from build123d import *

# Parameters (mm, degrees)
F0_R        = 7.5
F1_DEPTH    = 20
F0_W        = 45
F0_H        = 45
F2_DEPTH    = 5
F3_R        = 2.5
F4_DEPTH    = 25
F5_R        = 10
F5_R_2      = 7.5
F6_DEPTH    = 7
F7_W        = 8
F7_H        = 9.7702028193
F7_W_2      = 5
F7_H_2      = 4.5
F8_DEPTH    = 2
F9_T3_DEPTH = 70
F9_T5_DEPTH = 70


# Not quite as in the source:
# - a fillet or chamfer that OpenCascade refuses, or shapes differently, is made with other operations: its cross-section is extruded or revolved along the edge and cut away or added


with BuildPart() as f1:
    # F0 (on Front) → F1 (new body)
    with BuildSketch(Plane.XZ):
        with Locations((-2.8196598027, -8.5107027553)):
            Circle(F0_R)
    extrude(amount=F1_DEPTH)

    # F0 (on Front) → F2 (join)
    with BuildSketch(Plane.XZ):
        with Locations((-2.8196598027, -8.5107027553)):
            Rectangle(F0_W, F0_H)
        with Locations((-2.8196598027, -8.5107027553)):
            Circle(F0_R, mode=Mode.SUBTRACT)
    extrude(amount=F2_DEPTH)

    # F3 (on face) → F4 (cut)
    with BuildSketch(Plane.XZ.offset(5)):
        with Locations((12.1803401973, 7.9892972447)):
            Circle(F3_R)
        with Locations((-17.8196598027, 7.9892972447)):
            Circle(F3_R)
    extrude(amount=-F4_DEPTH, mode=Mode.SUBTRACT)

    # F5 (on face) → F6 (join)
    with BuildSketch(Plane.XZ.offset(20)):
        with Locations((-2.8196598027, -8.5107027553)):
            Circle(F5_R)
        with Locations((-2.8196598027, -8.5107027553)):
            Circle(F5_R_2, mode=Mode.SUBTRACT)
        with Locations((-2.8196598027, -8.5107027553)):
            Circle(F5_R_2)
    extrude(amount=F6_DEPTH)

    # F7 (on face) → F8 (cut)
    with BuildSketch(Plane.XZ.offset(27)):
        with Locations((-2.8196598027, -15.6458041649)):
            Rectangle(F7_W, F7_H)
        with Locations((-9.3196598027, -8.5107027553)):
            Rectangle(F7_W_2, F7_H_2)
        with Locations((-2.8196598027, -8.5107027553)):
            Rectangle(F7_W, F7_H_2)
        with Locations((3.6803401973, -8.5107027553)):
            Rectangle(F7_W_2, F7_H_2)
        with Locations((-2.8196598027, -1.3756013457)):
            Rectangle(F7_W, F7_H)
    extrude(amount=-F8_DEPTH, mode=Mode.SUBTRACT)

    # F9: fillet of radius 5 on 7 edges, made by hand

    # F9_s1 → F9_t2 (revolve)
    with BuildSketch(Plane.XY.offset(-8.5107027553)):
        with BuildLine():
            ThreePointArc((4.6803401973, -10), (6.1448062914, -6.4644660941), (9.6803401973, -5))
            Line((9.6803401973, -5), (4.6803401973, -5))
            Line((4.6803401973, -5), (4.6803401973, -10))
        make_face()
    revolve(axis=Axis((-2.8196598027, -5, -8.5107027553), (0, -1, 0)))

    # F9_s4 → F9_t3 (cut)
    with BuildSketch(Plane.YZ.offset(-37.8196598027)):
        with BuildLine():
            ThreePointArc((-5, 8.9892972447), (-3.5355339059, 12.5248311506), (0, 13.9892972447))
            Line((0, 13.9892972447), (-5, 13.9892972447))
            Line((-5, 13.9892972447), (-5, 8.9892972447))
        make_face()
        with BuildLine():
            ThreePointArc((-5, -26.0107027553), (-3.5355339059, -29.5462366612), (0, -31.0107027553))
            Line((0, -31.0107027553), (-5, -31.0107027553))
            Line((-5, -31.0107027553), (-5, -26.0107027553))
        make_face()
    extrude(amount=F9_T3_DEPTH, mode=Mode.SUBTRACT)

    # F9_s6 → F9_t5 (cut)
    with BuildSketch(Plane.XY.offset(-43.5107027553)):
        with BuildLine():
            ThreePointArc((14.6803401973, -5), (18.2158741033, -3.5355339059), (19.6803401973, 0))
            Line((19.6803401973, 0), (19.6803401973, -5))
            Line((19.6803401973, -5), (14.6803401973, -5))
        make_face()
        with BuildLine():
            ThreePointArc((-20.3196598027, -5), (-23.8551937086, -3.5355339059), (-25.3196598027, 0))
            Line((-25.3196598027, 0), (-25.3196598027, -5))
            Line((-25.3196598027, -5), (-20.3196598027, -5))
        make_face()
    extrude(amount=F9_T5_DEPTH, mode=Mode.SUBTRACT)

    # F9_s7 → F9_t8 (revolve, cut)
    with BuildSketch(Plane.XY.offset(7.9892972447)):
        with BuildLine():
            ThreePointArc((-10.3196598027, -5), (-13.8551937086, -3.5355339059), (-15.3196598027, 0))
            Line((-15.3196598027, 0), (-15.3196598027, -5))
            Line((-15.3196598027, -5), (-10.3196598027, -5))
        make_face()
    revolve(axis=Axis((-17.8196598027, -5, 7.9892972447), (0, -1, 0)), mode=Mode.SUBTRACT)

    # F9_s9 → F9_t10 (revolve, cut)
    with BuildSketch(Plane.XY.offset(7.9892972447)):
        with BuildLine():
            ThreePointArc((19.6803401973, -5), (16.1448062914, -3.5355339059), (14.6803401973, 0))
            Line((14.6803401973, 0), (14.6803401973, -5))
            Line((14.6803401973, -5), (19.6803401973, -5))
        make_face()
    revolve(axis=Axis((12.1803401973, -5, 7.9892972447), (0, -1, 0)), mode=Mode.SUBTRACT)

    # F10: fillet of radius 8 on 1 edges, made by hand

    # F10_s1 → F10_t2 (revolve, cut)
    with BuildSketch(Plane.XY.offset(-8.5107027553)):
        with BuildLine():
            ThreePointArc((7.1803401973, -25.8094750193), (6.5288094257, -22.6471973591), (4.6803401973, -20))
            Line((4.6803401973, -20), (7.1803401973, -20))
            Line((7.1803401973, -20), (7.1803401973, -25.8094750193))
        make_face()
    revolve(axis=Axis((-2.8196598027, -20, -8.5107027553), (0, -1, 0)), mode=Mode.SUBTRACT)


solid = f1.part
The listing builds one solid part. Answer for the finished solid, in the listing's coordinates (mm). A direction names the side the tool comes from. Round coordinates to 2 decimals unless told otherwise and drop trailing zeros. Order: outer loops, then holes, each group sorted by start corner. A loop starts at its lowest first (then second) coordinate and runs counter-clockwise, first axis right, second up. Notation, with made-up numbers: M 34,-18.75 L 61,-18.75 A13 cw 61,-5.75 Z; hole C 82,61.25 d4. An arc over 180 degrees is marked long. Answer in a Markdown table with one row per item. Add a question column.
1) Flat-ended cylindrical pins translate along their axes: pin 1 Ø10 at (x, y) = (-5, -14) entering from +Z; pin 2 Ø2 at (y, z) = (-26, -8) entering from +X; pin 3 Ø2 at (x, y) = (-9.5, -25.5) entering from -Z. Find the tip coordinate at first contact, or state that the pin passes through.
2) The part is cut by section A-A on y = -3. Determine the outline of the cut face in (x, z), plus the area to 3 significant figures.
3) Which of the six approach directions +Z, -Z, +X, -X, +Y, -Y give full straight-line access (tool end or side, diameter ignored) to faces 4 (the face through (1.18, -26, -14)), 5 (the face through (-12.82, -26.4, -8.35)), 6 (the face through (-9, -26, -6.261)), 7 (the face through (4.334, -14.93, -6.258))?
4) Consider line 1 along X through (y, z) = (-2.5, 10.5); line 2 along Y through (x, z) = (-5.5, -9); line 3 along Y through (x, z) = (-10, -12). Determine where each line is inside the solid, lowest interval first. Write a range as from..to.
5) The part is cut by section C-C on y = -18.5. Determine the outline of the cut face in (x, z), plus the area to 3 significant figures.
6) Determine the mould class of faces 1 (the face through (-23.82, -3.57, -8.83)), 2 (the face through (-11, -5, -20)), 3 (the face through (4, -26, -6.261)) for opening direction X: pulls with the +X half, pulls with the -X half, needs draft (parallel to the pull), parting line crosses it, or undercut.
7) The part is cut by section B-B on z = -22. Determine the outline of the cut face in (x, y).
8) The part is cut by section D-D on y = -5.75. Determine the outline of the cut face in (x, z).
Findings below:
| question | item | result |
|---|---|---|
| 1 | pin 1 | stops at z = -0.98 |
| 1 | pin 2 | stops at x = 7.18 |
| 1 | pin 3 | stops at z = -16.73 |
| 2 | outline | M -24.32,-30.01 L 18.68,-30.01 L 18.68,12.99 L -24.32,12.99 Z; hole C -17.82,7.99 d7; hole C 12.18,7.99 d7 |
| 2 | area | 1,770 mm² |
| 3 | face 4 | +Z, -Z, -Y |
| 3 | face 5 | -X, -Y |
| 3 | face 6 | -Y |
| 3 | face 7 | none |
| 4 | line 1 | x = -24.65..-19.75, -15.88..10.25, 14.12..19.01 |
| 4 | line 2 | y = -25..0 |
| 4 | line 3 | y = -27..-20.5, -7.86..0 |
| 5 | outline | C -2.82,-8.51 d15 |
| 5 | area | 177 mm² |
| 6 | face 1 | pulls with the -X half |
| 6 | face 2 | needs draft |
| 6 | face 3 | undercut |
| 7 | outline | M -25.32,0 A5 ccw -20.32,-5 L 14.68,-5 A5 ccw 19.68,0 Z |
| 8 | outline | C -2.82,-8.51 d19.73 |
